```python
from build123d import *

# Parameters (mm, degrees)
BOSS_EXTRUDE1_DEPTH = 6.35
SKETCH2_R           = 0.79375
CUT_EXTRUDE1_DEPTH  = 41.907013457


with BuildPart() as part:
    # Sketch1 → Boss-Extrude1 (new body)
    with BuildSketch(Plane.XY):
        with BuildLine():
            Line((0, 22.225), (0, 28.575))
            Line((0, 28.575), (13.126483451, 17.934493503))
            ThreePointArc((13.126483451, 17.934493503), (14.463585172, 16.87469493), (15.715448212, 15.715448212))
            Line((15.715448212, 15.715448212), (20.205576272, 20.205576272))
            Line((20.205576272, 20.205576272), (21.963427435, 3.399776512))
            ThreePointArc((21.963427435, 3.399776512), (22.159510371, 1.70491206), (22.225, 0))
            Line((22.225, 0), (28.575, 0))
            Line((28.575, 0), (17.934493503, -13.126483451))
            ThreePointArc((17.934493503, -13.126483451), (16.87469493, -14.463585172), (15.715448212, -15.715448212))
            Line((15.715448212, -15.715448212), (20.205576272, -20.205576272))
            Line((20.205576272, -20.205576272), (3.399776512, -21.963427435))
            ThreePointArc((3.399776512, -21.963427435), (1.70491206, -22.159510371), (0, -22.225))
            Line((0, -22.225), (0, -28.575))
            Line((0, -28.575), (-13.126483451, -17.934493503))
            ThreePointArc((-13.126483451, -17.934493503), (-14.463585172, -16.87469493), (-15.715448212, -15.715448212))
            Line((-15.715448212, -15.715448212), (-20.205576272, -20.205576272))
            Line((-20.205576272, -20.205576272), (-21.963427435, -3.399776512))
            ThreePointArc((-21.963427435, -3.399776512), (-22.159510371, -1.70491206), (-22.225, 0))
            Line((-22.225, 0), (-28.575, 0))
            Line((-28.575, 0), (-17.934493503, 13.126483451))
            ThreePointArc((-17.934493503, 13.126483451), (-16.87469493, 14.463585172), (-15.715448212, 15.715448212))
            Line((-15.715448212, 15.715448212), (-20.205576272, 20.205576272))
            Line((-20.205576272, 20.205576272), (-3.399776512, 21.963427435))
            ThreePointArc((-3.399776512, 21.963427435), (-1.70491206, 22.159510371), (0, 22.225))
        make_face()
    extrude(amount=BOSS_EXTRUDE1_DEPTH)

    # Sketch2 → Cut-Extrude1 (cut, through all)
    with BuildSketch(Plane.XY.offset(6.35)):
        Circle(SKETCH2_R)
    extrude(amount=-CUT_EXTRUDE1_DEPTH, mode=Mode.SUBTRACT)


solid = part.part
```
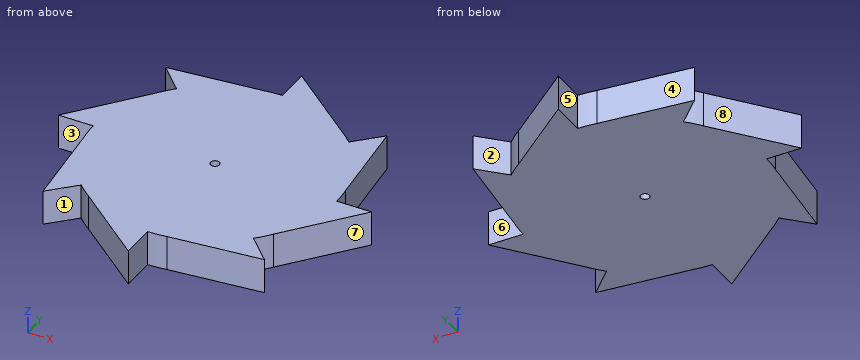
Could you check a few things on this model? Use its own coordinates, in mm. Face numbers are marked on the shaded views. A direction names the side the tool comes from. Give positions to 0.01 mm unless a question says otherwise; leave off trailing zeros. Loops run counter-clockwise (first coordinate to the right, second up) from the corner with the lowest first, then second, coordinate; pieces in that order, holes last. Notation, with made-up numbers: (29.25, 4) -> (86.25, 4) arc R30 cw to (86.25, 32) -> close; hole circle Ø5 at (-34.75, -20.5). An arc over 180 degrees is marked (long way). Put each result on its own line as item: value.
(1) I'm going to push flat-ended pins straight in: pin 1 Ø1 at (y, z) = (-15.5, 5) entering from +X; pin 2 Ø2 at (x, z) = (0, 3.5) entering from -Y (3 decimals); pin 3 Ø3 at (y, z) = (26.5, 4) entering from -X; pin 4 Ø10 at (x, y) = (16, -8.5) entering from -Z. Where does each tip first touch, or does it pass through?
Computed:
pin 1: x = 16.4
pin 2: y = -28.575
pin 3: x = 0
pin 4: z = 0
(2) Imagine slicing it at B-B on x = -19.5. Write out the boundary of the cut face in (y, z), plus the area to 3 significant figures.
Computed:
outline: (-19.5, 0) -> (11.2, 0) -> (11.2, 6.35) -> (-19.5, 6.35) -> close; (19.5, 0) -> (20.28, 0) -> (20.28, 6.35) -> (19.5, 6.35) -> close
area: 200 mm^2
(3) For the marked faces 5, 6, 7 and 8, which set-ups out of +Z, -Z, +X, -X, +Y, -Y let a thin tool reach every point of the face, with its end or its side?
Computed:
face 5: +Z, -Z, -X, +Y
face 6: +Z, -Z, +X, +Y
face 7: +Z, -Z, +X
face 8: +Z, -Z, -X
(4) Please list where these lines run through material, in increasing order: probe 1 along Y at (x, z) = (18, 3.5); probe 2 along Y at (x, z) = (-6.5, 5.5); probe 3 along X at (y, z) = (11, 3). Write a range as [from, to].
Computed:
probe 1: [-20.44, -18], [-13.05, 18]
probe 2: [-23.31, 21.64]
probe 3: [-19.66, 21.17]
(5) Imagine slicing it at C-C on y = 9. Write out the boundary of the cut face in (x, z), plus the area to 3 significant figures.
Computed:
outline: (-21.28, 0) -> (21.38, 0) -> (21.38, 6.35) -> (-21.28, 6.35) -> close
area: 271 mm^2
(6) Imagine slicing it at D-D on x = 6.5. Write out the boundary of the cut face in (y, z).
Computed:
outline: (-21.64, 0) -> (23.31, 0) -> (23.31, 6.35) -> (-21.64, 6.35) -> close
(7) Thinking about a two-plate mould opening in X: for the marked faces 1, 2, 3 and 4, which applies, pulls with the +X half, pulls with the -X half, needs draft (parallel to the pull), parting line crosses it, or undercut?
Computed:
face 1: undercut
face 2: undercut
face 3: needs draft
face 4: pulls with the -X half
